from build123d import *

# Parameters (mm, degrees)
SKETCH2_R           = 50
BOSS_EXTRUDE1_DEPTH = 35
SKETCH3_W           = 8
SKETCH3_H           = 35
CUT_EXTRUDE1_DEPTH  = 20
SKETCH4_R           = 3.5
CUT_EXTRUDE2_DEPTH  = 80
SKETCH5_R           = 3.5
CUT_EXTRUDE3_DEPTH  = 50
SKETCH6_R           = 3.5
CUT_EXTRUDE4_DEPTH  = 50
SKETCH8_W           = 14.038446545
SKETCH8_H           = 6.5
CUT_EXTRUDE5_DEPTH  = 15.5
SKETCH11_W          = 8
SKETCH11_H          = 6.5
BOSS_EXTRUDE2_DEPTH = 4.5
BOSS_EXTRUDE3_DEPTH = 15.5
BOSS_EXTRUDE4_DEPTH = 35
SKETCH18_R          = 3.5
CUT_EXTRUDE9_DEPTH  = 25
SKETCH19_R          = 3.5
CUT_EXTRUDE10_DEPTH = 25
SKETCH20_R          = 3.5
CUT_EXTRUDE11_DEPTH = 25
SKETCH21_W          = 5.1
SKETCH21_H          = 18.4
CUT_EXTRUDE12_DEPTH = 13
SKETCH23_W          = 5.1
SKETCH23_H          = 18.4
CUT_EXTRUDE13_DEPTH = 13
SKETCH22_W          = 5.1
SKETCH22_H          = 13.3
BOSS_EXTRUDE5_DEPTH = 7.9
CUT_EXTRUDE14_DEPTH = 8.5
SKETCH25_R          = 9
CUT_EXTRUDE15_DEPTH = 20


with BuildPart() as part:
    # Sketch2 → Boss-Extrude1 (new body)
    with BuildSketch(Plane.XY):
        Circle(SKETCH2_R)
    extrude(amount=BOSS_EXTRUDE1_DEPTH)

    # Sketch3 → Cut-Extrude1 (cut)
    with BuildSketch(Plane(origin=(0, 0, 0), x_dir=(-1, 0, 0), z_dir=(0, 0, -1))):
        with Locations((0, 21.5)):
            Rectangle(SKETCH3_W, SKETCH3_H)
        Polygon((31.774990748, -22.964101615), (35.774990748, -16.035898385), (5.464101615, 1.464101615), (1.464101615, -5.464101615), align=None)
        Polygon((-35.774990748, -16.035898385), (-31.774990748, -22.964101615), (-1.464101615, -5.464101615), (-5.464101615, 1.464101615), align=None)
    extrude(amount=-CUT_EXTRUDE1_DEPTH, mode=Mode.SUBTRACT)

    # Sketch4 → Cut-Extrude2 (cut)
    with BuildSketch(Plane(origin=(-3.464101615, -2, 0), x_dir=(0, 0, 1), z_dir=(-0.866025404, -0.5, 0))):
        with Locations((10, 0)):
            Circle(SKETCH4_R)
    extrude(amount=CUT_EXTRUDE2_DEPTH, mode=Mode.SUBTRACT)

    # Sketch5 → Cut-Extrude3 (cut)
    with BuildSketch(Plane(origin=(0, 4, 0), x_dir=(1, 0, 0), z_dir=(0, 1, 0))):
        with Locations((0, -10)):
            Circle(SKETCH5_R)
    extrude(amount=CUT_EXTRUDE3_DEPTH, mode=Mode.SUBTRACT)

    # Sketch6 → Cut-Extrude4 (cut)
    with BuildSketch(Plane(origin=(3.464101615, -2, 0), x_dir=(0, 0, -1), z_dir=(0.866025404, -0.5, 0))):
        with Locations((-10, 0)):
            Circle(SKETCH6_R)
    extrude(amount=CUT_EXTRUDE4_DEPTH, mode=Mode.SUBTRACT)

    # Sketch8 → Cut-Extrude5 (cut)
    with BuildSketch(Plane(origin=(0, 0, 0), x_dir=(-1, 0, 0), z_dir=(0, 0, -1))):
        Polygon((-32.971083956, -10.892407408), (-25.951860683, -23.050058746), (-20.322695558, -19.800058746), (-27.341918831, -7.642407408), align=None)
        with Locations((0.033217181, 30.75)):
            Rectangle(SKETCH8_W, SKETCH8_H)
        Polygon((27.30870165, -7.699941254), (32.937866774, -10.949941254), (25.918643502, -23.107592592), (20.289478377, -19.857592592), align=None)
    extrude(amount=-CUT_EXTRUDE5_DEPTH, mode=Mode.SUBTRACT)

    # Sketch11 → Boss-Extrude2 (add)
    with BuildSketch(Plane(origin=(0, 0, 20), x_dir=(-1, 0, 0), z_dir=(0, 0, -1))):
        with Locations((0, 30.75)):
            Rectangle(SKETCH11_W, SKETCH11_H)
        Polygon((25.815698604, -10.285898385), (31.444863729, -13.535898385), (27.444863729, -20.464101615), (21.815698604, -17.214101615), align=None)
        Polygon((-21.815698604, -17.214101615), (-27.444863729, -20.464101615), (-31.444863729, -13.535898385), (-25.815698604, -10.285898385), align=None)
    extrude(amount=BOSS_EXTRUDE2_DEPTH)

    # Sketch12 → Boss-Extrude3 (add)
    with BuildSketch(Plane(origin=(0, 0, 15.5), x_dir=(-1, 0, 0), z_dir=(0, 0, -1))):
        Polygon((-6.986006091, 32.1), (7.052440454, 32.1), (7.052440454, 34), (4, 34), (4, 39), (-4, 39), (-4, 34), (-6.986006091, 34), align=None)
        Polygon((25.918643502, -23.107592592), (27.444863729, -20.464101615), (31.774990748, -22.964101615), (35.774990748, -16.035898385), (31.444863729, -13.535898385), (32.937866774, -10.949941254), (31.292418507, -9.999941254), (24.273195235, -22.157592592), align=None)
        Polygon((-32.971083956, -10.892407408), (-31.444863729, -13.535898385), (-35.774990748, -16.035898385), (-31.774990748, -22.964101615), (-27.444863729, -20.464101615), (-25.951860683, -23.050058746), (-24.306412416, -22.100058746), (-31.325635688, -9.942407408), align=None)
    extrude(amount=BOSS_EXTRUDE3_DEPTH)

    # Sketch17 → Boss-Extrude4 (add)
    with BuildSketch(Plane(origin=(0, 0, 0), x_dir=(-1, 0, 0), z_dir=(0, 0, -1))):
        Polygon((-5.842787082, 32.897450406), (-5.842787082, 43.509531182), (5.727819383, 43.509531182), (5.754751517, 32.897450406), align=None)
        Polygon((31.411421312, -11.388723161), (25.612652013, -21.432486209), (34.816449619, -26.715202685), (40.601752851, -16.69476355), align=None)
        Polygon((-25.568634231, -21.508727245), (-31.36740353, -11.464964197), (-40.544269002, -16.794328497), (-34.75896577, -26.814767633), align=None)
    extrude(amount=-BOSS_EXTRUDE4_DEPTH)

    # Sketch18 → Cut-Extrude9 (cut, symmetric)
    with BuildSketch(Plane(origin=(-37.680359311, -21.754765591, 0), x_dir=(0, 0, 1), z_dir=(-0.866025404, -0.5, 0))):
        with Locations((10, 0)):
            Circle(SKETCH18_R)
    extrude(amount=CUT_EXTRUDE9_DEPTH, both=True, mode=Mode.SUBTRACT)

    # Sketch19 → Cut-Extrude10 (cut, symmetric)
    with BuildSketch(Plane(origin=(37.680359311, -21.754765591, 0), x_dir=(0, 0, -1), z_dir=(0.866025404, -0.5, 0))):
        with Locations((-10, 0)):
            Circle(SKETCH19_R)
    extrude(amount=CUT_EXTRUDE10_DEPTH, both=True, mode=Mode.SUBTRACT)

    # Sketch20 → Cut-Extrude11 (cut, symmetric)
    with BuildSketch(Plane(origin=(0, 43.509531182, 0), x_dir=(1, 0, 0), z_dir=(0, 1, 0))):
        with Locations((0, -10)):
            Circle(SKETCH20_R)
    extrude(amount=CUT_EXTRUDE11_DEPTH, both=True, mode=Mode.SUBTRACT)

    # Sketch21 → Cut-Extrude12 (cut)
    with BuildSketch(Plane(origin=(0, 0, 0), x_dir=(-1, 0, 0), z_dir=(0, 0, -1))):
        with Locations((6.55, 13.2)):
            Rectangle(SKETCH21_W, SKETCH21_H)
    extrude(amount=-CUT_EXTRUDE12_DEPTH, mode=Mode.SUBTRACT)

    # Sketch23 → Cut-Extrude13 (cut)
    with BuildSketch(Plane(origin=(0, 0, 0), x_dir=(-1, 0, 0), z_dir=(0, 0, -1))):
        with Locations((6.55, 13.2)):
            Rectangle(SKETCH23_W, SKETCH23_H)
        Polygon((-1.085898385, -9.880831174), (1.464101615, -5.464101615), (17.398969045, -14.664101615), (14.848969045, -19.080831174), align=None)
        Polygon((-8.014101615, 5.880831174), (-5.464101615, 1.464101615), (-21.398969045, -7.735898385), (-23.948969045, -3.319168826), align=None)
    extrude(amount=-CUT_EXTRUDE13_DEPTH, mode=Mode.SUBTRACT)

    # Sketch22 → Boss-Extrude5 (add)
    with BuildSketch(Plane(origin=(0, 0, 0), x_dir=(-1, 0, 0), z_dir=(0, 0, -1))):
        with Locations((6.55, 10.65)):
            Rectangle(SKETCH22_W, SKETCH22_H)
        Polygon((-1.085898385, -9.880831174), (1.464101615, -5.464101615), (12.982239485, -12.114101615), (10.432239485, -16.530831174), align=None)
        Polygon((-8.014101615, 5.880831174), (-5.464101615, 1.464101615), (-16.982239485, -5.185898385), (-19.532239485, -0.769168826), align=None)
    extrude(amount=-BOSS_EXTRUDE5_DEPTH)

    # Sketch24 → Cut-Extrude14 (cut)
    with BuildSketch(Plane.XY.offset(35)):
        with BuildLine():
            Line((0.831568399, -1), (1.11810064, -0.999925477))
            ThreePointArc((1.11810064, -0.999925477), (0.535186435, 1.401276375), (-1.5, 0))
            ThreePointArc((-1.5, 0), (-1.401274891, -0.535190321), (-1.118095094, -0.999931678))
            Line((-1.118095094, -0.999931678), (-0.831313787, -1))
            Line((-0.831313787, -1), (0.831568399, -1))
        make_face()
    extrude(amount=-CUT_EXTRUDE14_DEPTH, mode=Mode.SUBTRACT)

    # Sketch25 → Cut-Extrude15 (cut)
    with BuildSketch(Plane(origin=(0, 0, 0), x_dir=(-1, 0, 0), z_dir=(0, 0, -1))):
        Circle(SKETCH25_R)
    extrude(amount=-CUT_EXTRUDE15_DEPTH, mode=Mode.SUBTRACT)


solid = part.part
Verification items for the finished model (mm, model axes). A direction names the side the tool comes from. Give positions to 0.01 mm unless a question says otherwise; leave off trailing zeros. Write each loop counter-clockwise with the first axis right and the second up, starting at its lowest first coordinate (ties: lowest second). Pieces come first, ordered by that corner, then holes. Notation, with made-up numbers: (86, 21.25) - (134, 21.25) arc R19 ccw to (134, 34.25) - close; hole circle Ø10 at (66.25, 25). An arc over 180 degrees is marked (long way). Answer as CSV lines item,"result". Start each with the question number.
1. Sectioned sample at C-C (z = 10). Count the separate pieces of the cut face and the enclosed holes in it, then the cut area to 3 significant figures.
2. Depth check by flat-ended pin: pin 1 (2 mm diameter, centred on y = 20, z = 3.5, fed in from +X); pin 2 (12 mm diameter, centred on y = -26.5, z = 13, fed in from -X); pin 3 (3.5 mm diameter, centred on x = 0, y = 0, fed in from -Z). Enter the tip coordinate at first touch or a pass-through.
3. Sectioned sample at A-A (y = 40). Record the boundary of the cut face in (x, z).
4. Set-up check for faces 3 (the face through (-9.1, 15, 9)), 4 (the face through (-0.759, 40.927, 13.417)), 5 (the face through (0, 0, 26.5)), 6 (the face through (6, 27.5, 8)): record each of +Z, -Z, +X, -X, +Y, -Y from which the full face is reachable in a straight line by a thin tool's end or side.
5. Thickness scan on line 1 (Z direction, x = 0, y = 45); line 2 (X direction, y = -16.5, z = 12.5); line 3 (Y direction, x = 0, z = 29.75). Record the ranges inside material, lowest first.
6. Sectioned sample at D-D (y = -30.5). Record the boundary of the cut face in (x, z), then the cut area to 3 significant figures.
7. Sectioned sample at B-B (z = 29). Record the boundary of the cut face in (x, y), then the cut area to 3 significant figures.
8. Draft check along X on faces 1 (the face through (-23.788, -13.798, 17.782)), 2 (the face through (-4, 20, 14)). Enter one of: pulls with the +X half, pulls with the -X half, needs draft (parallel to the pull), parting line crosses it, or undercut.
Derived:
1,separate pieces,"3"
1,enclosed holes,"0"
1,area,"6,330 mm²"
2,pin 1,"x = 46.25"
2,pin 2,"x = -45.6"
2,pin 3,"z = 20"
3,outline,"(-30, 0) - (30, 0) - (30, 35) - (-30, 35) - close; hole circle Ø7 at (0, 10)"
4,face 3,"none"
4,face 4,"+Y"
4,face 5,"+Z"
4,face 6,"-Z"
5,line 1,"0 to 6.5, 13.5 to 35"
5,line 2,"-47.2 to -33.48, -20.58 to -16.34, -10.38 to 20.58, 33.48 to 47.2"
5,line 3,"-50 to -1, 1.5 to 50"
6,outline,"(-39.62, 0) - (39.62, 0) - (39.62, 35) - (-39.62, 35) - close"
6,area,"2,770 mm²"
7,outline,"circle Ø100 at (0, 0); hole (-1.12, -1) - (-0.83, -1) - (0.83, -1) - (1.12, -1) arc R1.5 ccw (long way) to start"
7,area,"7,850 mm²"
8,face 1,"undercut"
8,face 2,"undercut"
